Verification items for this drawing (mm, ordinates from the low corner). Give positions to 0.01 mm unless a question says otherwise; leave off trailing zeros. Write each loop counter-clockwise with the first axis right and the second up, starting at its lowest first coordinate (ties: lowest second). Pieces come first, ordered by that corner, then holes. Notation, with made-up numbers: (-39.75, -18) -> (-2.75, -18) arc R30 cw to (-2.75, 20) -> close; hole circle Ø1 at (68, 89). An arc over 180 degrees is marked (long way). Write item = value, one per line.
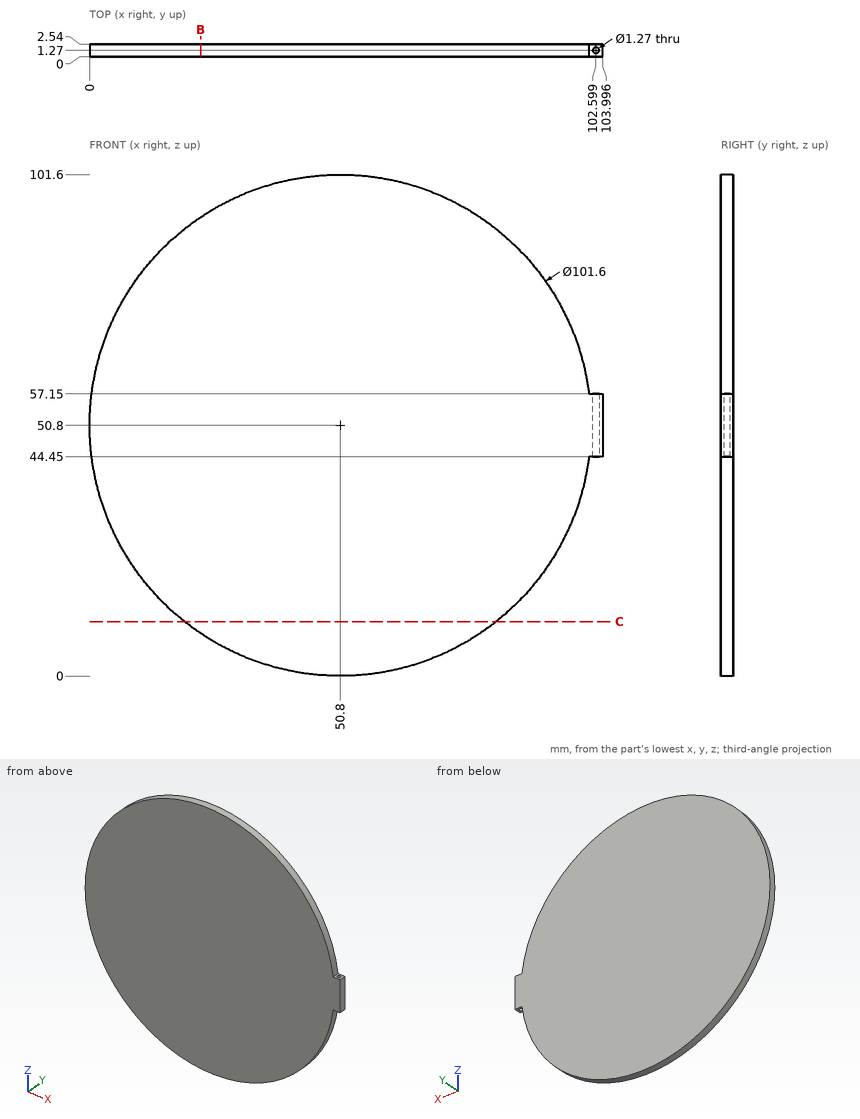
Item 1: Sectioned sample at B-B on x = 22.5. Record the cut outline in (y, z).
Response values:
outline = (0, 8.61) -> (2.54, 8.61) -> (2.54, 92.99) -> (0, 92.99) -> close
Item 2: Sectioned sample at C-C on z = 11. Record the cut outline in (x, y), then the cut area to 3 significant figures.
Response values:
outline = (19.23, 0) -> (82.37, 0) -> (82.37, 2.54) -> (19.23, 2.54) -> close
area = 160 mm^2
Item 3: Go/stop test with flat-tipped pins: P1, Ø0.8, axis at x = 103, y = 1, coming from the -Z side; P2, Ø1.3, axis at x = 102, y = 0.5, coming from the +Z side. Record where each tip stops, or that it passes through.
Response values:
P1 = 44.45
P2 = 57.15
Item 4: Material ranges on line 1 (X direction, y = 1.25, z = 37); line 2 (Z direction, x = 19, y = 1.75) (1 decimal); line 3 (X direction, y = 1.6, z = 26) (1 decimal), recorded low to high.
Response values:
line_1 = 1.91 to 99.69
line_2 = 11.2 to 90.4
line_3 = 6.5 to 95.1
